For this review, use the dimensioned drawing (mm, ordinates from the lowest corner) and the shaded views. Coordinates: 2 decimals unless noted, no trailing zeros. Order: outer loops, then holes, each group sorted by start corner. A loop starts at its lowest first (then second) coordinate and runs counter-clockwise, first axis right, second up. Notation, with made-up numbers: M 21,-26.5 L 55,-26.5 A7 ccw 55,-20.5 Z; hole C -1.75,-2 d6. An arc over 180 degrees is marked long. Answer in a Markdown table with one row per item.
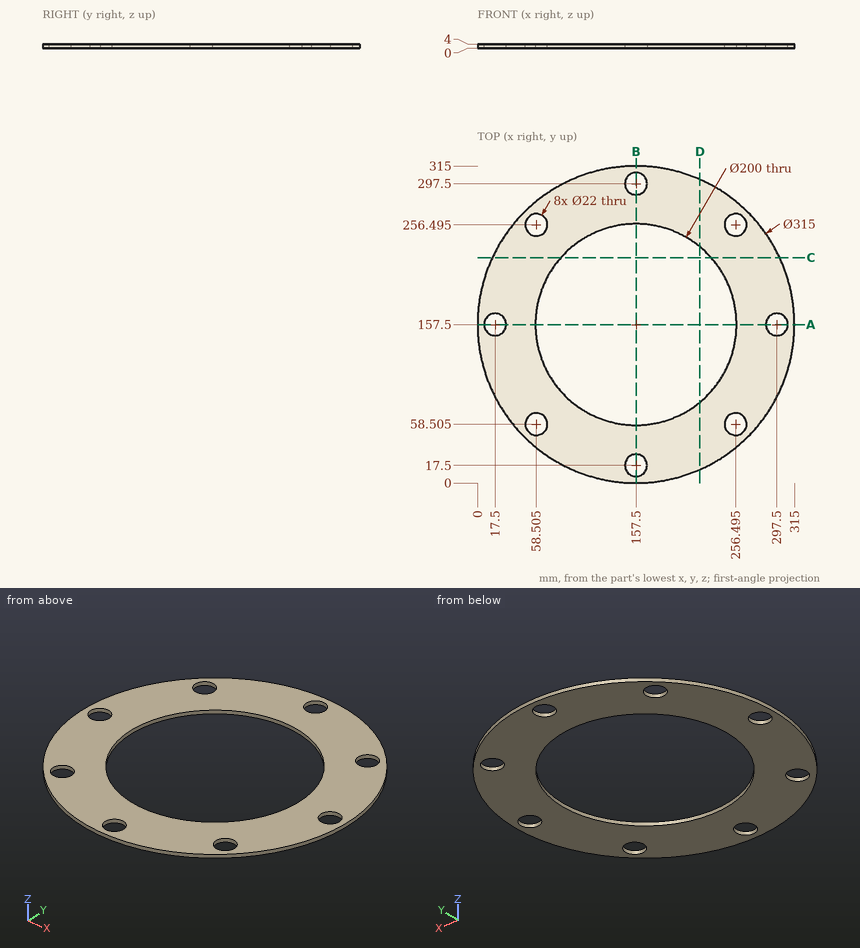
(1) Add section C-C, the plane y = 224. Give the boundary of the cut face in (x, z), and give its area (3 significant figures).
Return value:
| item | result |
|---|---|
| outline | M 14.73,0 L 82.82,0 L 82.82,4 L 14.73,4 Z; M 232.18,0 L 300.27,0 L 300.27,4 L 232.18,4 Z |
| area | 545 mm2 |
(2) For line 1 along Y through (x, z) = (157.5, 1); line 2 along X through (y, z) = (165, 3.3); line 3 along Y through (x, z) = (21, 0.2) (1 decimal), list the stretches that pass through material, from the lowest coordinate up. Write a range as from..to.
Return value:
| item | result |
|---|---|
| line 1 | y = 0..6.5, 28.5..57.5, 257.5..286.5, 308.5..315 |
| line 2 | x = 0.18..9.45, 25.55..57.78, 257.22..289.45, 305.55..314.82 |
| line 3 | y = 78.9..147.1, 167.9..236.1 |
(3) Add section A-A, the plane y = 157.5. Give the boundary of the cut face in (x, z), and give its area (3 significant figures).
Return value:
| item | result |
|---|---|
| outline | M 0,0 L 6.5,0 L 6.5,4 L 0,4 Z; M 28.5,0 L 57.5,0 L 57.5,4 L 28.5,4 Z; M 257.5,0 L 286.5,0 L 286.5,4 L 257.5,4 Z; M 308.5,0 L 315,0 L 315,4 L 308.5,4 Z |
| area | 284 mm2 |
(4) Add section D-D, the plane x = 221. Give the boundary of the cut face in (y, z).
Return value:
| item | result |
|---|---|
| outline | M 13.37,0 L 80.25,0 L 80.25,4 L 13.37,4 Z; M 234.75,0 L 301.63,0 L 301.63,4 L 234.75,4 Z |
(5) Insertion check: pin 1 Ø17.5 at (x, y) = (58.51, 256.49) entering from +Z; pin 2 Ø1.5 at (y, z) = (36, 1.5) entering from +X; pin 3 Ø1.5 at (y, z) = (217.5, 3.5) entering from -X; pin 4 Ø1 at (x, z) = (99.5, 3) entering from +Y. Each pin has a flat end and moves straight along its axis. Give the tip position at first contact, or say it passes through.
Return value:
| item | result |
|---|---|
| pin 1 | passes through |
| pin 2 | stops at x = 258.62 |
| pin 3 | stops at x = 11.57 |
| pin 4 | stops at y = 304.13 |
